```python
from build123d import *

# Parameters (mm, degrees)
F0_R     = 8.4832662773
F1_DEPTH = 91.44
F2_W     = 59.8430555439
F2_H     = 102.967698127
F3_DEPTH = 57.658
F4_DEPTH = 25.4


# Not quite as in the source:
# - the program builds the solid bodies; features that only make, move or delete a surface that nothing else refers to are left out


with BuildPart() as f1:
    # F0 (on Front) → F1 (new body)
    with BuildSketch(Plane.XZ):
        with BuildLine():
            Line((20.1094433592, -48.163229742), (20.1094433592, 54.4155371868))
            ThreePointArc((20.1094433592, 54.4155371868), (0.0972339361, 74.7201513345), (-20.1103836136, 54.6100027859))
            Line((-20.1103836136, 54.6100027859), (-20.1103836136, -48.3576953411))
            ThreePointArc((-20.1103836136, -48.3576953411), (-0.0972339361, -28.2475467925), (20.1094433592, -48.163229742))
        make_face()
        with Locations((0, 54.6100027859)):
            Circle(F0_R, mode=Mode.SUBTRACT)
        with BuildLine():
            Line((20.1094433592, -48.5521609402), (20.1094433592, -48.163229742))
            ThreePointArc((20.1094433592, -48.163229742), (-0.0972339361, -28.2475467925), (-20.1103836136, -48.3576953411))
            ThreePointArc((-20.1103836136, -48.3576953411), (-0.0972339361, -68.4678438897), (20.1094433592, -48.5521609402))
        make_face()
        with Locations((0, -48.3576953411)):
            Circle(F0_R, mode=Mode.SUBTRACT)
    extrude(amount=F1_DEPTH)

    # F2 (on face) → F3 (cut)
    with BuildSketch(Plane(origin=(-20.1103836136, 0, 0), x_dir=(0, -1, 0), z_dir=(-1, 0, 0))):
        with Locations((45.72, 106.0938518494)):
            Rectangle(F2_W, F2_H)
        with Locations((45.72, 3.1261537224)):
            Rectangle(F2_W, F2_H)
    extrude(amount=-F3_DEPTH, mode=Mode.SUBTRACT)

    # F0 (on Front) → F4 (join)
    with BuildSketch(Plane.XZ):
        with BuildLine():
            Line((20.1094433592, -48.163229742), (20.1094433592, 54.4155371868))
            ThreePointArc((20.1094433592, 54.4155371868), (0.0972339361, 74.7201513345), (-20.1103836136, 54.6100027859))
            Line((-20.1103836136, 54.6100027859), (-20.1103836136, -48.3576953411))
            ThreePointArc((-20.1103836136, -48.3576953411), (-0.0972339361, -28.2475467925), (20.1094433592, -48.163229742))
        make_face()
        with Locations((0, 54.6100027859)):
            Circle(F0_R, mode=Mode.SUBTRACT)
        with BuildLine():
            Line((20.1094433592, -48.5521609402), (20.1094433592, -48.163229742))
            ThreePointArc((20.1094433592, -48.163229742), (-0.0972339361, -28.2475467925), (-20.1103836136, -48.3576953411))
            ThreePointArc((-20.1103836136, -48.3576953411), (-0.0972339361, -68.4678438897), (20.1094433592, -48.5521609402))
        make_face()
        with Locations((0, -48.3576953411)):
            Circle(F0_R, mode=Mode.SUBTRACT)
        with BuildLine():
            ThreePointArc((20.1103836136, -48.3576953411), (20.1101485486, -48.260461405), (20.1094433592, -48.163229742))
            Line((20.1094433592, -48.163229742), (20.1094433592, -48.5521609402))
            ThreePointArc((20.1094433592, -48.5521609402), (20.1101485486, -48.4549292772), (20.1103836136, -48.3576953411))
        make_face()
    extrude(amount=F4_DEPTH)


solid = f1.part
```
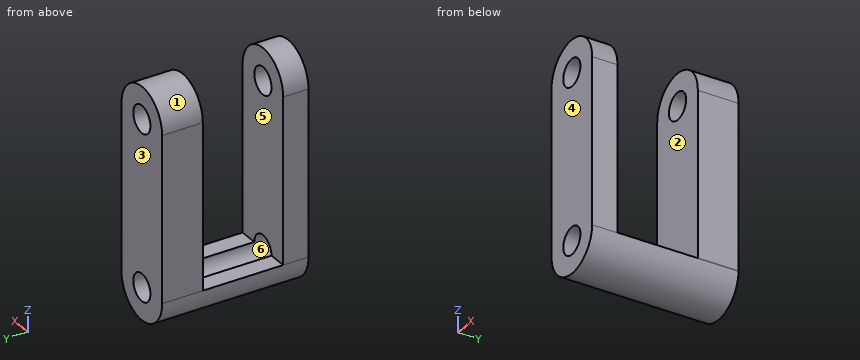
The listing builds one solid part. Answer for the finished solid, in the listing's coordinates (mm). Face numbers are marked on the shaded views. A direction names the side the tool comes from. Give positions to 0.01 mm unless a question says otherwise; leave off trailing zeros. Write each loop counter-clockwise with the first axis right and the second up, starting at its lowest first coordinate (ties: lowest second). Pieces come first, ordered by that corner, then holes. Notation, with made-up numbers: (13, 24) -> (34, 24) arc R5 cw to (34, 30) -> close; hole circle Ø11 at (88.5, -5). An arc over 180 degrees is marked (long way). Use one line per item in the form item = value.
1) Straight lines are drawn through the part: probe 1 along Z at (x, y) = (0, -8.75); probe 2 along Y at (x, z) = (18, -43); probe 3 along X at (y, z) = (-41, -49). For each, find the intervals that lie inside material, in ascending order.
Result:
probe_1 = -68.47 to -56.84, -39.87 to 46.13, 63.09 to 74.72
probe_2 = -91.44 to -75.64, -25.4 to 0
probe_3 = -20.1 to -8.46, 8.46 to 20.1
2) For a pull along Y with two mould halves and no side action, classify the marked faces 1, 2, 3 and 4 as +Y half, -Y half, draft (parallel to the pull), parting line (faces both ways), or undercut.
Result:
face_1 = draft
face_2 = undercut
face_3 = +Y half
face_4 = -Y half
3) Each of these flat-tipped pins is pushed along its axis until it touches: P1, Ø10, axis at y = -56.5, z = -40, coming from the -X side; P2, Ø9.5, axis at x = -17, y = -57, coming from the +Z side; P3, Ø8, axis at x = -10.5, y = -59, coming from the -Z side; P4, Ø5, axis at x = 12, y = -16, coming from the -Z side. Where does it stop, or does it pass through?
Result:
P1 = through
P2 = -48.36
P3 = -67.39
P4 = -66.08
4) Section B-B on z = 10.5 is taken. Write down the section's boundary in (x, y).
Result:
outline = (-20.11, -91.44) -> (20.11, -91.44) -> (20.11, -75.64) -> (-20.11, -75.64) -> close; (-20.11, -25.4) -> (20.11, -25.4) -> (20.11, 0) -> (-20.11, 0) -> close
5) Section C-C on y = -21.5 is taken. Write down the section's boundary in (x, z), plus the area to 3 significant figures.
Result:
outline = (-20.11, -48.36) arc R20.11 ccw to (20.11, -48.55) arc R20.11 ccw to (20.11, -48.16) -> (20.11, 54.42) arc R20.11 ccw (long way) to (-20.11, 54.61) -> close; hole circle Ø16.97 at (0, -48.36); hole circle Ø16.97 at (0, 54.61)
area = 4,960 mm²
6) A tool of negligible diameter and unlimited length cuts with its end or side. For the marked faces 5 and 6, from which of +Z, -Z, +X, -X, +Y, -Y can it reach the whole face along a straight path? Write none if from no direction.
Result:
face_5 = +Z, +X, -X
face_6 = +Y, -Y
7) Section A-A on x = 0 is taken. Write down the section's boundary in (y, z), plus the area to 3 significant figures.
Result:
outline = (-91.44, -68.47) -> (0, -68.47) -> (0, -56.84) -> (-91.44, -56.84) -> close; (-91.44, -39.87) -> (-75.64, -39.87) -> (-75.64, 46.13) -> (-91.44, 46.13) -> close; (-91.44, 63.09) -> (-75.64, 63.09) -> (-75.64, 74.72) -> (-91.44, 74.72) -> close; (-25.4, -39.87) -> (0, -39.87) -> (0, 46.13) -> (-25.4, 46.13) -> close; (-25.4, 63.09) -> (0, 63.09) -> (0, 74.72) -> (-25.4, 74.72) -> close
area = 5,090 mm²
8) Section D-D on z = 50 is taken. Write down the section's boundary in (x, y).
Result:
outline = (-20.11, -91.44) -> (-7.12, -91.44) -> (-7.12, -75.64) -> (-20.11, -75.64) -> close; (-20.11, -25.4) -> (-7.12, -25.4) -> (-7.12, 0) -> (-20.11, 0) -> close; (7.12, -91.44) -> (20.11, -91.44) -> (20.11, -75.64) -> (7.12, -75.64) -> close; (7.12, -25.4) -> (20.11, -25.4) -> (20.11, 0) -> (7.12, 0) -> close
